from build123d import *

# Parameters (mm, degrees)
SKETCH_1_W          = 140
SKETCH_1_H          = 140
SKETCH_1_R          = 1.55
EXTRUDE_1_DEPTH     = 3
SKETCH_2_R          = 1.55
SKETCH_2_W          = 3
SKETCH_2_H          = 25
CUT_EXTRUDE_1_DEPTH = 100.040395799
SKETCH_3_R          = 5
SKETCH_3_R_2        = 1.55
EXTRUDE_2_DEPTH     = 3
CUT_EXTRUDE_START   = -10
SKETCH_4_R          = 1.55
CUT_EXTRUDE_2_DEPTH = 10


with BuildPart() as part:
    # 草圖1 → 填料-伸長1 (new body)
    with BuildSketch(Plane.XY):
        Rectangle(SKETCH_1_W, SKETCH_1_H)
        with Locations((-60, 60)):
            Circle(SKETCH_1_R, mode=Mode.SUBTRACT)
        with Locations((60, 60)):
            Circle(SKETCH_1_R, mode=Mode.SUBTRACT)
        with Locations((60, -60)):
            Circle(SKETCH_1_R, mode=Mode.SUBTRACT)
        with Locations((-60, -60)):
            Circle(SKETCH_1_R, mode=Mode.SUBTRACT)
    extrude(amount=EXTRUDE_1_DEPTH)

    # 草圖2 → 除料-伸長1 (cut, through all)
    with BuildSketch(Plane.XY.offset(3)):
        with Locations((-12.25, 62.5)):
            Circle(SKETCH_2_R)
        with Locations((12.25, 62.5)):
            Circle(SKETCH_2_R)
        with Locations((-12.25, 7.5)):
            Circle(SKETCH_2_R)
        with Locations((12.25, 7.5)):
            Circle(SKETCH_2_R)
        with Locations((-60, -30)):
            Rectangle(SKETCH_2_W, SKETCH_2_H)
        with Locations((-60, 30)):
            Rectangle(SKETCH_2_W, SKETCH_2_H)
        with Locations((-20, -30)):
            Rectangle(SKETCH_2_W, SKETCH_2_H)
        with Locations((-20, 30)):
            Rectangle(SKETCH_2_W, SKETCH_2_H)
        with Locations((20, 30)):
            Rectangle(SKETCH_2_W, SKETCH_2_H)
        with Locations((20, -30)):
            Rectangle(SKETCH_2_W, SKETCH_2_H)
        with Locations((60, -30)):
            Rectangle(SKETCH_2_W, SKETCH_2_H)
        with Locations((60, 30)):
            Rectangle(SKETCH_2_W, SKETCH_2_H)
    extrude(amount=-CUT_EXTRUDE_1_DEPTH, mode=Mode.SUBTRACT)

    # 草圖3 → 填料-伸長2 (add)
    # profile 1 of 4: a face of its own
    with BuildSketch(Plane.XY.offset(3)):
        with BuildLine():
            Line((-79.393398282, 100.606601718), (-48.786796564, 70))
            Line((-48.786796564, 70), (-70, 70))
            Line((-70, 70), (-70, 48.786796564))
            Line((-70, 48.786796564), (-100.606601718, 79.393398282))
            ThreePointArc((-100.606601718, 79.393398282), (-100.606601718, 100.606601718), (-79.393398282, 100.606601718))
        make_face()
        with Locations((-90, 90)):
            Circle(SKETCH_3_R, mode=Mode.SUBTRACT)
        with Locations((-81, 90)):
            Circle(SKETCH_3_R_2, mode=Mode.SUBTRACT)
        with Locations((-90, 98)):
            Circle(SKETCH_3_R_2, mode=Mode.SUBTRACT)
        with Locations(Location((-99, 90, 0), (0, 0, 180))):
            Circle(SKETCH_3_R_2, mode=Mode.SUBTRACT)
        with Locations(Location((-90, 82, 0), (0, 0, 180))):
            Circle(SKETCH_3_R_2, mode=Mode.SUBTRACT)
    # profile 2 of 4: a face of its own
    with BuildSketch(Plane.XY.offset(3)):
        with BuildLine():
            Line((48.786796564, 70), (70, 70))
            Line((70, 70), (70, 48.786796564))
            Line((70, 48.786796564), (100.606601718, 79.393398282))
            ThreePointArc((100.606601718, 79.393398282), (100.606601718, 100.606601718), (79.393398282, 100.606601718))
            Line((79.393398282, 100.606601718), (48.786796564, 70))
        make_face()
        with Locations(Location((81, 90, 0), (0, 0, 180))):
            Circle(SKETCH_3_R_2, mode=Mode.SUBTRACT)
        with Locations(Location((90, 90, 0), (0, 0, 180))):
            Circle(SKETCH_3_R, mode=Mode.SUBTRACT)
        with Locations((90, 82)):
            Circle(SKETCH_3_R_2, mode=Mode.SUBTRACT)
        with Locations(Location((90, 98, 0), (0, 0, 180))):
            Circle(SKETCH_3_R_2, mode=Mode.SUBTRACT)
        with Locations((99, 90)):
            Circle(SKETCH_3_R_2, mode=Mode.SUBTRACT)
    # profile 3 of 4: a face of its own
    with BuildSketch(Plane.XY.offset(3)):
        with BuildLine():
            Line((-48.786796564, -70), (-70, -70))
            Line((-70, -70), (-70, -48.786796564))
            Line((-70, -48.786796564), (-100.606601718, -79.393398282))
            ThreePointArc((-100.606601718, -79.393398282), (-100.606601718, -100.606601718), (-79.393398282, -100.606601718))
            Line((-79.393398282, -100.606601718), (-48.786796564, -70))
        make_face()
        with Locations((-90, -82)):
            Circle(SKETCH_3_R_2, mode=Mode.SUBTRACT)
        with Locations(Location((-90, -90, 0), (0, 0, 180))):
            Circle(SKETCH_3_R, mode=Mode.SUBTRACT)
        with Locations(Location((-81, -90, 0), (0, 0, 180))):
            Circle(SKETCH_3_R_2, mode=Mode.SUBTRACT)
        with Locations(Location((-90, -98, 0), (0, 0, 180))):
            Circle(SKETCH_3_R_2, mode=Mode.SUBTRACT)
        with Locations((-99, -90)):
            Circle(SKETCH_3_R_2, mode=Mode.SUBTRACT)
    # profile 4 of 4: a face of its own
    with BuildSketch(Plane.XY.offset(3)):
        with BuildLine():
            Line((79.393398282, -100.606601718), (48.786796564, -70))
            Line((48.786796564, -70), (70, -70))
            Line((70, -70), (70, -48.786796564))
            Line((70, -48.786796564), (100.606601718, -79.393398282))
            ThreePointArc((100.606601718, -79.393398282), (100.606601718, -100.606601718), (79.393398282, -100.606601718))
        make_face()
        with Locations(Location((90, -82, 0), (0, 0, 180))):
            Circle(SKETCH_3_R_2, mode=Mode.SUBTRACT)
        with Locations((90, -90)):
            Circle(SKETCH_3_R, mode=Mode.SUBTRACT)
        with Locations((81, -90)):
            Circle(SKETCH_3_R_2, mode=Mode.SUBTRACT)
        with Locations((90, -98)):
            Circle(SKETCH_3_R_2, mode=Mode.SUBTRACT)
        with Locations(Location((99, -90, 0), (0, 0, 180))):
            Circle(SKETCH_3_R_2, mode=Mode.SUBTRACT)
    extrude(amount=-EXTRUDE_2_DEPTH)

    # 草圖4 → 除料-伸長2 (cut)
    with BuildSketch(Plane(origin=(0, 0, 0), x_dir=(-1, 0, 0), z_dir=(0, 0, -1)).offset(CUT_EXTRUDE_START)):
        with Locations((-70, 70)):
            Circle(SKETCH_4_R)
        with BuildLine():
            Line((-70, 48.786796564), (-65, 48.786796564))
            Line((-65, 48.786796564), (-48.786796564, 65))
            Line((-48.786796564, 65), (-48.786796564, 70))
            Line((-48.786796564, 70), (48.786796564, 70))
            Line((48.786796564, 70), (79.393398282, 100.606601718))
            ThreePointArc((79.393398282, 100.606601718), (100.606601718, 100.606601718), (100.606601718, 79.393398282))
            Line((100.606601718, 79.393398282), (70, 48.786796564))
            Line((70, 48.786796564), (70, -48.786796564))
            Line((70, -48.786796564), (100.606601718, -79.393398282))
            ThreePointArc((100.606601718, -79.393398282), (100.606601718, -100.606601718), (79.393398282, -100.606601718))
            Line((79.393398282, -100.606601718), (48.786796564, -70))
            Line((48.786796564, -70), (-48.786796564, -70))
            Line((-48.786796564, -70), (-79.393398282, -100.606601718))
            ThreePointArc((-79.393398282, -100.606601718), (-100.606601718, -100.606601718), (-100.606601718, -79.393398282))
            Line((-100.606601718, -79.393398282), (-70, -48.786796564))
            Line((-70, -48.786796564), (-70, 48.786796564))
        make_face()
    extrude(amount=CUT_EXTRUDE_2_DEPTH, mode=Mode.SUBTRACT)


solid = part.part
Work out the finished part from the listing and answer in its coordinate system (mm). Coordinates: 2 decimals unless noted, no trailing zeros. Write each loop counter-clockwise with the first axis right and the second up, starting at its lowest first coordinate (ties: lowest second). Pieces come first, ordered by that corner, then holes. Notation, with made-up numbers: M -7.5,82 L 49.5,82 A7 ccw 49.5,92 Z; hole C 11.25,39 d8. An arc over 180 degrees is marked long. Use one line per item in the form item = value. Start each with the question number.
1. Straight lines are drawn through the part: probe 1 along Y at (x, z) = (90, 2.2); probe 2 along X at (y, z) = (90, 1.7); probe 3 along Y at (x, z) = (90.5, 2.35). For each, find the intervals that lie inside material, in ascending order. Write a range as from..to.
2. The mould has two halves that part along Y. Classify faces 1 (the face through (68, 48.787, 2)), 2 (the face through (85.381, 91.915, 1.521)), 3 (the face through (48.787, 67, 2)), 4 (the face through (61.478, 60.466, 1.479)): released by +Y, released by -Y, zero draft, split by the parting line, or undercut.
3. The part is cut by section A-A (z = 1.35). Give the vertices of the cut face in (x, y).
4. The part is cut by section D-D (y = 90). Give the vertices of the cut face in (x, z).
5. The part is cut by section B-B (y = 82). Give the vertices of the cut face in (x, z).
6. Each of these flat-tipped pins is pushed along its axis until it touches: P1, Ø4, axis at x = 99, y = 90, coming from the -Z side; P2, Ø3, axis at x = 81, y = 90, coming from the -Z side; P3, Ø1.5, axis at y = 61, z = 0.5, coming from the -X side; P4, Ø1, axis at x = 65, z = 1.5, coming from the +Y side. Where does it stop, or does it pass through?
7. The part is cut by section C-C (x = 90). Give the vertices of the cut face in (y, z), plus the area to 3 significant figures.
Evaluation:
q1.probe_1 = 68.79..80.45, 83.55..85, 95..96.45, 99.55..105
q1.probe_2 = 68.79..79.45, 82.55..85, 95..97.45, 100.55..105
q1.probe_3 = 69.29..80.53, 83.47..85.03, 94.97..96.53, 99.47..104.99
q2.face_1 = released by -Y
q2.face_2 = undercut
q2.face_3 = zero draft
q2.face_4 = undercut
q3.outline = M 48.79,65 L 65,48.79 L 70,48.79 L 100.61,79.39 A15 ccw 79.39,100.61 L 48.79,70 Z; hole C 60,60 d3.1; hole C 70,70 d3.1; hole C 81,90 d3.1; hole C 90,90 d10; hole C 90,82 d3.1; hole C 90,98 d3.1; hole C 99,90 d3.1
q4.outline = M 68.79,0 L 79.45,0 L 79.45,3 L 68.79,3 Z; M 82.55,0 L 85,0 L 85,3 L 82.55,3 Z; M 95,0 L 97.45,0 L 97.45,3 L 95,3 Z; M 100.55,0 L 105,0 L 105,3 L 100.55,3 Z
q5.outline = M 60.79,0 L 88.45,0 L 88.45,3 L 60.79,3 Z; M 91.55,0 L 102.69,0 L 102.69,3 L 91.55,3 Z
q6.P1 = 0
q6.P2 = through
q6.P3 = 52.04
q6.P4 = 86.71
q7.outline = M 68.79,0 L 80.45,0 L 80.45,3 L 68.79,3 Z; M 83.55,0 L 85,0 L 85,3 L 83.55,3 Z; M 95,0 L 96.45,0 L 96.45,3 L 95,3 Z; M 99.55,0 L 105,0 L 105,3 L 99.55,3 Z
q7.area = 60.0 mm^2
